from build123d import *

# Parameters (mm, degrees)
F0_W     = 665
F0_H     = 535
F1_DEPTH = 105
F2_W     = 635
F2_H     = 505
F3_DEPTH = 90
F5_D     = 12
F6_W     = 635
F6_H     = 15
F7_DEPTH = 60
F8_SIZE2 = 15
F8_SIZE  = 60
F9_R     = 27
F11_D    = 8


with BuildPart() as f1:
    # F0 (on Front) → F1 (new body)
    with BuildSketch(Plane.XZ):
        with Locations((332.5, 267.5)):
            Rectangle(F0_W, F0_H)
    extrude(amount=-F1_DEPTH)

    # F2 (on face) → F3 (cut, through all)
    with BuildSketch(Plane(origin=(0, 105, 0), x_dir=(-1, 0, 0), z_dir=(0, 1, 0))):
        with Locations((-332.5, 267.5)):
            Rectangle(F2_W, F2_H)
    extrude(amount=-F3_DEPTH, mode=Mode.SUBTRACT)

    # F5 (through all)
    with Locations(Plane.YZ.offset(665)):
        with Locations((57.5, 57.5)):
            Hole(F5_D / 2)

    # F6 (on face) → F7 (cut)
    with BuildSketch(Plane(origin=(0, 105, 0), x_dir=(-1, 0, 0), z_dir=(0, 1, 0))):
        with Locations((-332.5, 7.5)):
            Rectangle(F6_W, F6_H)
    extrude(amount=-F7_DEPTH, mode=Mode.SUBTRACT)

    # F8
    f8_edges = [f1.edges().sort_by_distance(p)[0] for p in [
        (657.5, 105, 0),
        (7.5, 105, 0),
    ]]
    f8_side = f1.faces().sort_by_distance((332.5, 25.478723, 0))[0]
    chamfer(f8_edges, length=F8_SIZE, length2=F8_SIZE2, reference=f8_side)

    # F9
    f9_edges = [f1.edges().sort_by_distance(p)[0] for p in [
        (657.5, 105, 15),
        (7.5, 105, 15),
    ]]
    fillet(f9_edges, radius=F9_R)

    # F11 (through all)
    with Locations(Plane(origin=(0, 0, 0), x_dir=(0, -1, 0), z_dir=(-1, 0, 0))):
        with Locations((-80, 30)):
            Hole(F11_D / 2)


solid = f1.part
Design review of the part built by this model. Coordinates are the model's own, in mm. A direction names the side the tool comes from. Give positions to 0.01 mm unless a question says otherwise; leave off trailing zeros. Loops run counter-clockwise (first coordinate to the right, second up) from the corner with the lowest first, then second, coordinate; pieces in that order, holes last. Notation, with made-up numbers: (85.25, 24.25) -> (99.25, 24.25) arc R21 cw to (99.25, 33.25) -> close; hole circle Ø11 at (36.25, 30). An arc over 180 degrees is marked (long way). One line per question, with ' | ' between items. Start each with the question number.
(1) We need section C-C (x = 600.5). State the section outline as (y, z) points, and give its area (4 significant figures).
(2) We need section B-B (z = 88.5). State the section outline as (x, y) points, and give its area (3 significant figures).
(3) For faces 1 (the face through (337, 61, 520)), 2 (the face through (337, 45, 8)), 3 (the face through (7, 65, 5)), list the 3-axis set-ups (+Z, -Z, +X, -X, +Y, -Y) from which the entire face can be reached by the end or side of a thin tool; tool diameter is ignored.
(4) For line 1 (X direction, y = 78.5, z = 488); line 2 (Z direction, x = 201, y = 42); line 3 (Z direction, x = 451, y = 68), list the stretches that pass through material, from the lowest coordinate up.
(5) We need section A-A (y = 24.5). State the section outline as (x, z) points, and give its area (3 significant figures).
(6) Insertion check: P1, Ø7, axis at y = 80, z = 30, coming from the +X side; P2, Ø6, axis at x = 207, y = 84, coming from the -Z side; P3, Ø3, axis at x = 229, z = 285, coming from the +Y side; P4, Ø16.5, axis at x = 389, z = 10.5, coming from the +Y side. Each pin has a flat end and moves straight along its axis. Give the tip position at first contact, or say it passes through.
(7) Draft analysis for pull direction X (two halves, no side actions). For faces 4 (the face through (665, 52, 264)), 5 (the face through (337, 30, 15)), 6 (the face through (657, 65, 5)), state which applies: +X half, -X half, draft (parallel to the pull), parting line (faces both ways), or undercut.
The answers:
1) outline: (0, 0) -> (45, 0) -> (45, 15) -> (15, 15) -> (15, 520) -> (105, 520) -> (105, 535) -> (0, 535) -> close | area: 9,825 mm^2
2) outline: (0, 0) -> (665, 0) -> (665, 105) -> (650, 105) -> (650, 15) -> (15, 15) -> (15, 105) -> (0, 105) -> close | area: 12,700 mm^2
3) face 1: +Y | face 2: -Z, +Y | face 3: -Z, +X, -X, +Y
4) line 1: x = 0 to 15, 650 to 665 | line 2: z = 0 to 15, 520 to 535 | line 3: z = 520 to 535
5) outline: (0, 0) -> (665, 0) -> (665, 535) -> (0, 535) -> close; hole (15, 15) -> (650, 15) -> (650, 520) -> (15, 520) -> close | area: 35,100 mm^2
6) P1: passes through | P2: stops at z = 520 | P3: stops at y = 15 | P4: stops at y = 45
7) face 4: +X half | face 5: undercut | face 6: draft
